from build123d import *

# Parameters (mm, degrees)
F0_R     = 11.1125
F1_DEPTH = 25.4


with BuildPart() as f1:
    # F0 (on Top) → F1 (new body)
    with BuildSketch(Plane.XY):
        Circle(F0_R)
        with BuildLine():
            ThreePointArc((6.1483610621, -1.5875), (-6.35, 0), (6.1483610621, 1.5875))
            Line((6.1483610621, 1.5875), (7.9375, 1.5875))
            Line((7.9375, 1.5875), (7.9375, -1.5875))
            Line((7.9375, -1.5875), (6.1483610621, -1.5875))
        make_face(mode=Mode.SUBTRACT)
        with BuildLine():
            ThreePointArc((6.1483610621, 1.5875), (6.2993885713, 0.8001272573), (6.35, 0))
            ThreePointArc((6.35, 0), (6.2993885713, -0.8001272573), (6.1483610621, -1.5875))
            Line((6.1483610621, -1.5875), (7.9375, -1.5875))
            Line((7.9375, -1.5875), (7.9375, 1.5875))
            Line((7.9375, 1.5875), (6.1483610621, 1.5875))
        make_face()
        with BuildLine():
            ThreePointArc((6.1483610621, -1.5875), (6.2993885713, -0.8001272573), (6.35, 0))
            ThreePointArc((6.35, 0), (6.2993885713, 0.8001272573), (6.1483610621, 1.5875))
            Line((6.1483610621, 1.5875), (4.7625, 1.5875))
            Line((4.7625, 1.5875), (4.7625, -1.5875))
            Line((4.7625, -1.5875), (6.1483610621, -1.5875))
        make_face()
    extrude(amount=F1_DEPTH)


solid = f1.part
Geometry: final body of the model. Coordinates: model frame, mm. A direction names the side the tool comes from. Round coordinates to 2 decimals unless told otherwise and drop trailing zeros. Order: outer loops, then holes, each group sorted by start corner. A loop starts at its lowest first (then second) coordinate and runs counter-clockwise, first axis right, second up. Notation, with made-up numbers: (18.5, 16) -> (22.5, 16) arc R19 ccw to (22.5, 34) -> close; hole circle Ø8 at (22, -37). An arc over 180 degrees is marked (long way). Put each result on its own line as item: value. Start each with the question number.
Q1. First-contact query: pin 1 (6 mm diameter, centred on y = -5, z = 10, fed in from +X); pin 2 (1.5 mm diameter, centred on x = 5.5, z = 18.5, fed in from -Y); pin 3 (4 mm diameter, centred on x = -6.5, y = -5, fed in from -Z); pin 4 (2 mm diameter, centred on y = -4.5, z = 21, fed in from +X). Flat tips, straight axial feed; report the tip coordinate or a pass-through.
Q2. Section B-B on x = 0. Return the cut outline in (y, z), and give its area (3 significant figures).
Q3. Pull-direction query (X, two-part tool) for faces 3 (the flat face through (5, 1.588, 13)), 4 (the flat face through (5, 0, 25.4)), 5 (the cylindrical face through (10.6, 3.34, 12.52)); classes: +X half, -X half, draft (parallel to the pull), parting line (faces both ways), or undercut.
Q4. Section A-A on y = 0. Return the cut outline in (x, z), and give its area (3 significant figures).
Q5. Section D-D on x = 8. Return the cut outline in (y, z), and give its area (3 significant figures).
Q6. Line query: probe 1 along Y at (x, z) = (0, 5.5); probe 2 along X at (y, z) = (-3, 5); probe 3 along X at (y, z) = (5.25, 12.5). Output: solid intervals per line, ascending.
Q7. Reachability of faces 1 (the flat face through (5, 0, 0)), 2 (the flat face through (5, -1.588, 13)) from +Z, -Z, +X, -X, +Y, -Y: full face, straight path, thin tool, end or side. Return the list, or none.
Ans:
1. pin 1: stops at x = 10.93
1. pin 2: stops at y = -10.05
1. pin 3: stops at z = 0
1. pin 4: stops at x = 10.55
2. outline: (-11.11, 0) -> (-6.35, 0) -> (-6.35, 25.4) -> (-11.11, 25.4) -> close; (6.35, 0) -> (11.11, 0) -> (11.11, 25.4) -> (6.35, 25.4) -> close
2. area: 242 mm2
3. face 3: undercut
3. face 4: draft
3. face 5: parting line
4. outline: (-11.11, 0) -> (-6.35, 0) -> (-6.35, 25.4) -> (-11.11, 25.4) -> close; (4.76, 0) -> (11.11, 0) -> (11.11, 25.4) -> (4.76, 25.4) -> close
4. area: 282 mm2
5. outline: (-7.71, 0) -> (7.71, 0) -> (7.71, 25.4) -> (-7.71, 25.4) -> close
5. area: 392 mm2
6. probe 1: y = -11.11 to -6.35, 6.35 to 11.11
6. probe 2: x = -10.7 to -5.6, 5.6 to 10.7
6. probe 3: x = -9.79 to -3.57, 3.57 to 9.79
7. face 1: -Z, +X, -X, +Y, -Y
7. face 2: +Z, -Z
